Check sheet for the modelled part. Datum: model origin and axes. Units: mm. Give positions to 0.01 mm unless a question says otherwise; leave off trailing zeros. Write each loop counter-clockwise with the first axis right and the second up, starting at its lowest first coordinate (ties: lowest second). Pieces come first, ordered by that corner, then holes. Notation, with made-up numbers: M -10.75,-9 L -2.75,-9 A20 cw -2.75,10 Z; hole C 34.5,67 d10. An arc over 180 degrees is marked long. Use CSV: the item, a comma, the result in double quotes. Start each with the question number.
1. Cross-section at C-C, the plane z = 4.3. Enter the section's corners in (x, y), and give its area (3 significant figures).
2. Scan lines: line 1 (Y direction, x = 5.5, z = 2.7); line 2 (X direction, y = -8.25, z = 2.5); line 3 (Y direction, x = 7.5, z = 4.55). Record each from-to range of solid material in increasing order.
3. Cross-section at B-B, the plane y = 0. Enter the section's corners in (x, z).
4. Cross-section at A-A, the plane x = 5.5. Enter the section's corners in (y, z).
5. Cross-section at D-D, the plane x = 8.25. Enter the section's corners in (y, z), and give its area (3 significant figures).
6. Mould release check, pull along Y, two halves, no side actions. Record for faces 1 (the face through (0, -10, 2)), 2 (the face through (5.85, -8.56, 2.46)), 3 (the face through (12.5, 0, 2)): +Y half, -Y half, draft (parallel to the pull), parting line (faces both ways), or undercut.
from build123d import *

# Parameters (mm, degrees)
F0_W     = 25
F0_H     = 20
F1_DEPTH = 5
F3_D     = 6.6
F3_DEPTH = 10
F3_TIP   = 1.9828400428
F4_R     = 2
F6_D     = 3.2
F6_DEPTH = 6
F6_TIP   = 0.9613769904


with BuildPart() as f1:
    # F0 (on Top) → F1 (new body)
    with BuildSketch(Plane.XY):
        Rectangle(F0_W, F0_H)
    extrude(amount=F1_DEPTH)

    # F3
    with Locations(Plane.XY.offset(5)):
        with Locations((5.5, 0)):
            Hole(F3_D / 2, depth=F3_DEPTH)
            with Locations((0, 0, -(F3_DEPTH + F3_TIP / 2))):  # 118° drill point
                Cone(0, F3_D / 2, F3_TIP, mode=Mode.SUBTRACT)

    # F4
    f4_edges = [f1.edges().sort_by_distance(p)[0] for p in [
        (-12.5, -10, 2.5),
        (-12.5, 10, 2.5),
        (12.5, -10, 2.5),
        (12.5, 10, 2.5),
    ]]
    fillet(f4_edges, radius=F4_R)

    # F6
    with Locations(Plane.XY.offset(5)):
        with Locations((5.5, 7), (5.5, -7)):
            Hole(F6_D / 2, depth=F6_DEPTH)
            with Locations((0, 0, -(F6_DEPTH + F6_TIP / 2))):  # 118° drill point
                Cone(0, F6_D / 2, F6_TIP, mode=Mode.SUBTRACT)


solid = f1.part
Worked answers:
1,outline,"M -12.5,-8 A2 ccw -10.5,-10 L 10.5,-10 A2 ccw 12.5,-8 L 12.5,8 A2 ccw 10.5,10 L -10.5,10 A2 ccw -12.5,8 Z; hole C 5.5,0 d6.6; hole C 5.5,-7 d3.2; hole C 5.5,7 d3.2"
1,area,"446 mm^2"
2,line 1,"y = -10 to -8.6, -5.4 to -3.3, 3.3 to 5.4, 8.6 to 10"
2,line 2,"x = -12.48 to 4.5, 6.5 to 12.48"
2,line 3,"y = -10 to -2.62, 2.62 to 10"
3,outline,"M -12.5,0 L 2.2,0 L 2.2,5 L -12.5,5 Z; M 8.8,0 L 12.5,0 L 12.5,5 L 8.8,5 Z"
4,outline,"M -10,0 L -8.6,0 L -8.6,5 L -10,5 Z; M -5.4,0 L -3.3,0 L -3.3,5 L -5.4,5 Z; M 3.3,0 L 5.4,0 L 5.4,5 L 3.3,5 Z; M 8.6,0 L 10,0 L 10,5 L 8.6,5 Z"
5,outline,"M -10,0 L -1.82,0 L -1.82,5 L -10,5 Z; M 1.82,0 L 10,0 L 10,5 L 1.82,5 Z"
5,area,"81.8 mm^2"
6,face 1,"-Y half"
6,face 2,"undercut"
6,face 3,"draft"
